The figure shows three views and two pictorial views of one solid part (mm, origin at its lowest corner). Answer the questions. Coordinates: 2 decimals unless noted, no trailing zeros. Write each loop counter-clockwise with the first axis right and the second up, starting at its lowest first coordinate (ties: lowest second). Pieces come first, ordered by that corner, then holes. Notation, with made-up numbers: (-2.75, 54.5) - (54.25, 54.5) arc R15 ccw to (54.25, 83.5) - close; hole circle Ø5 at (-34, 21). An arc over 180 degrees is marked (long way). Use a Markdown table: item, result. Add a question column.
(1) The part is cut by section D-D, the plane z = 16.5. Give the vertices of the cut face in (x, y).
(2) The part is cut by section B-B, the plane y = 4.8. Give the vertices of the cut face in (x, z).
(3) Find the intervals of material crossed by line 1 (X direction, y = 2.55, z = 2); line 2 (Z direction, x = 9.5, y = 3.2); line 3 (Z direction, x = 22.25, y = 1.85), in increasing order. Write a range as from..to.
(4) The part is cut by section C-C, the plane x = 14.5. Give the vertices of the cut face in (y, z).
(5) Given pin 1 Ø3 at (y, z) = (4, 51) entering from +X; pin 2 Ø1 at (y, z) = (3, 51) entering from -X; pin 3 Ø1.8 at (x, y) = (2.5, 2) entering from +Z; pin 4 Ø1.2 at (x, z) = (25.5, 2) entering from -Y, each flat-ended and moving along its own axis, determine where each tip first touches the part or whether it passes through.
(6) For a pull along Z with two mould halves and no side action, classify the marked faces 1, 2 and 3 as released by +Z, released by -Z, zero draft, split by the parting line, or undercut.
(7) The part is cut by section A-A, the plane z = 42.5. Give the vertices of the cut face in (x, y), then the cut area to 3 significant figures.
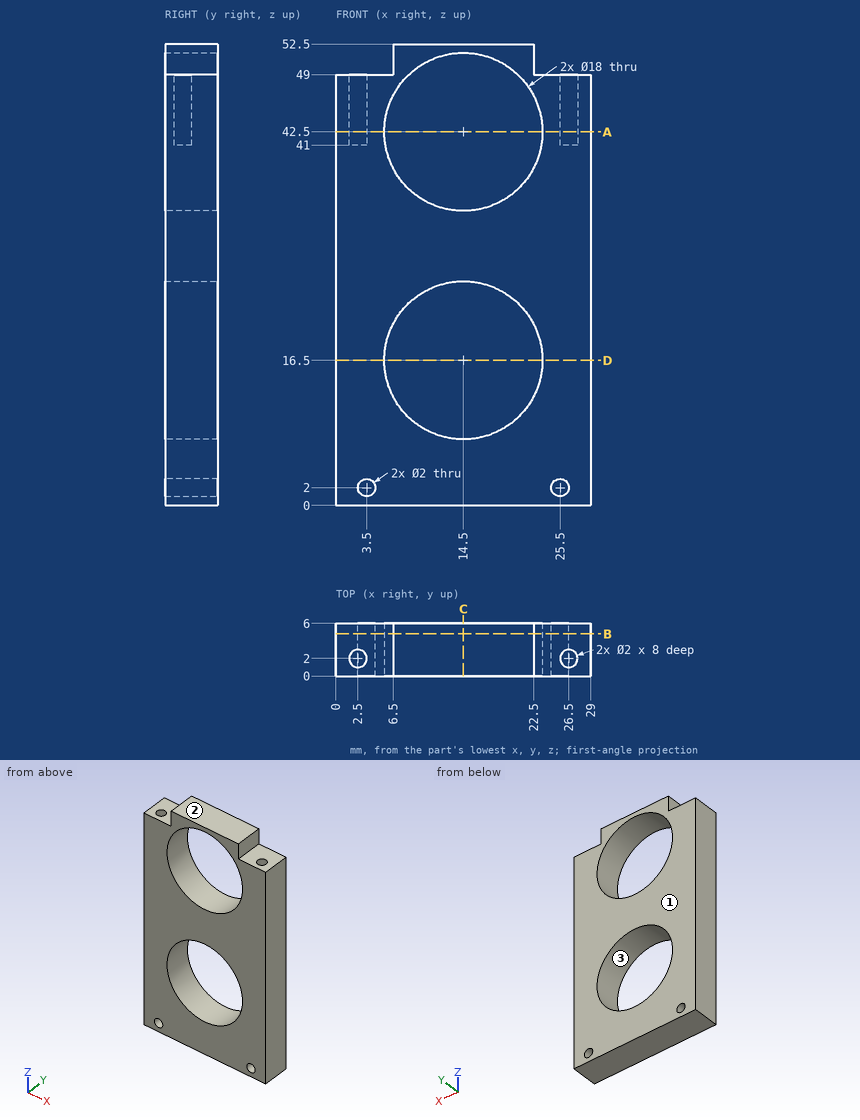
Model answer:
| question | item | result |
|---|---|---|
| 1 | outline | (0, 0) - (5.5, 0) - (5.5, 6) - (0, 6) - close; (23.5, 0) - (29, 0) - (29, 6) - (23.5, 6) - close |
| 2 | outline | (0, 0) - (29, 0) - (29, 49) - (22.5, 49) - (22.5, 52.5) - (6.5, 52.5) - (6.5, 49) - (0, 49) - close; hole circle Ø2 at (3.5, 2); hole circle Ø18 at (14.5, 16.5); hole circle Ø18 at (14.5, 42.5); hole circle Ø2 at (25.5, 2) |
| 3 | line 1 | 0..2.5, 4.5..24.5, 26.5..29 |
| 3 | line 2 | 0..9.02, 23.98..35.02, 49.98..52.5 |
| 3 | line 3 | 0..11.92, 21.08..37.92, 47.08..52.5 |
| 4 | outline | (0, 0) - (6, 0) - (6, 7.5) - (0, 7.5) - close; (0, 25.5) - (6, 25.5) - (6, 33.5) - (0, 33.5) - close; (0, 51.5) - (6, 51.5) - (6, 52.5) - (0, 52.5) - close |
| 5 | pin 1 | x = 22.5 |
| 5 | pin 2 | x = 6.5 |
| 5 | pin 3 | z = 41 |
| 5 | pin 4 | through |
| 6 | face 1 | zero draft |
| 6 | face 2 | released by +Z |
| 6 | face 3 | undercut |
| 7 | outline | (0, 0) - (5.5, 0) - (5.5, 6) - (0, 6) - close; (23.5, 0) - (29, 0) - (29, 6) - (23.5, 6) - close; hole circle Ø2 at (2.5, 2); hole circle Ø2 at (26.5, 2) |
| 7 | area | 59.7 mm^2 |
